Build history of the part. All positions in model axes, mm. A direction names the side the tool comes from. Give positions to 0.01 mm unless a question says otherwise; leave off trailing zeros. Order: outer loops, then holes, each group sorted by start corner. A loop starts at its lowest first (then second) coordinate and runs counter-clockwise, first axis right, second up. Notation, with made-up numbers: (41, 25) - (100, 25) arc R32 ccw to (100, 62) - close; hole circle Ø1 at (-38, 74). An arc over 180 degrees is marked (long way). One line per item, written item: value.
```python
from build123d import *

# Parameters (mm, degrees)
BOSS_EXTRUDE1_DEPTH     = 21.5
BOSS_EXTRUDE2_DEPTH     = 6
CHAMFER1_SIZE           = 1.5
SKETCH2_W               = 4.6
SKETCH2_H               = 18
CUT_EXTRUDE1_DEPTH      = 4.5000001
CUT_EXTRUDE1_DEPTH_BACK = 4.5000001
SKETCH3_R               = 1.6
CUT_EXTRUDE2_DEPTH      = 16
CHAMFER2_SIZE           = 0.5
SKETCH4_R               = 1.6
CUT_EXTRUDE3_DEPTH      = 7.0000001
CUT_EXTRUDE3_DEPTH_BACK = 7.0000001
SKETCH6_R               = 3
CUT_EXTRUDE4_DEPTH      = 2
CUT_EXTRUDE5_DEPTH      = 2
BOSS_EXTRUDE3_START     = -4.1
SKETCH8_R               = 1.6
BOSS_EXTRUDE3_DEPTH     = 3.5
BOSS_EXTRUDE4_DEPTH     = 9
BOSS_EXTRUDE5_DEPTH     = 9
CUT_EXTRUDE6_DEPTH      = 2
SKETCH13_W              = 5.8
SKETCH13_H              = 3
CUT_EXTRUDE8_DEPTH      = 18.5


with BuildPart() as part:
    # Sketch1 → Boss-Extrude1 (new body, symmetric)
    with BuildSketch(Plane.XY):
        with BuildLine():
            Line((-4.873397172, 3.5), (4.873397172, 3.5))
            ThreePointArc((4.873397172, 3.5), (6, 0), (4.873397172, -3.5))
            Line((4.873397172, -3.5), (-4.873397172, -3.5))
            ThreePointArc((-4.873397172, -3.5), (-6, 0), (-4.873397172, 3.5))
        make_face()
    extrude(amount=BOSS_EXTRUDE1_DEPTH, both=True)

    # Sketch5 → Boss-Extrude2 (add, symmetric)
    with BuildSketch(Plane(origin=(0, 0, 0), x_dir=(0, 0, -1), z_dir=(1, 0, 0))):
        with BuildLine():
            Line((-1.936491673, 3.5), (1.936491673, 3.5))
            ThreePointArc((1.936491673, 3.5), (4, 0), (1.936491673, -3.5))
            Line((1.936491673, -3.5), (-1.936491673, -3.5))
            ThreePointArc((-1.936491673, -3.5), (-4, 0), (-1.936491673, 3.5))
        make_face()
    extrude(amount=BOSS_EXTRUDE2_DEPTH, both=True)

    # Chamfer1
    chamfer1_edges = [part.edges().sort_by_distance(p)[0] for p in [
        (-6, 0, 21.5),
        (6, 0, 21.5),
        (-6, 0, -21.5),
        (6, 0, -21.5),
    ]]
    chamfer(chamfer1_edges, length=CHAMFER1_SIZE)

    # Sketch2 → Cut-Extrude1 (cut, two sides)
    with BuildSketch(Plane(origin=(0, 0, 0), x_dir=(1, 0, 0), z_dir=(0, 1, 0))) as cut_extrude1_sk:
        Rectangle(SKETCH2_W, SKETCH2_H)
    extrude(amount=CUT_EXTRUDE1_DEPTH, mode=Mode.SUBTRACT)
    extrude(cut_extrude1_sk.sketch, amount=-CUT_EXTRUDE1_DEPTH_BACK, mode=Mode.SUBTRACT)

    # Sketch3 → Cut-Extrude2 (cut)
    with BuildSketch(Plane.XY.offset(21.5)):
        Circle(SKETCH3_R)
    cut_extrude2 = extrude(amount=-CUT_EXTRUDE2_DEPTH, mode=Mode.SUBTRACT)

    # Mirror2: Cut-Extrude2 across plane
    add(cut_extrude2.mirror(Plane.XY), mode=Mode.SUBTRACT)

    # Chamfer2
    chamfer2_edges = [part.edges().sort_by_distance(p)[0] for p in [
        (-1.6, 0, 21.5),
        (-1.6, 0, -21.5),
    ]]
    chamfer(chamfer2_edges, length=CHAMFER2_SIZE)

    # Sketch4 → Cut-Extrude3 (cut, two sides)
    with BuildSketch(Plane(origin=(0, 0, 0), x_dir=(0, 0, -1), z_dir=(1, 0, 0))) as cut_extrude3_sk:
        Circle(SKETCH4_R)
    extrude(amount=CUT_EXTRUDE3_DEPTH, mode=Mode.SUBTRACT)
    extrude(cut_extrude3_sk.sketch, amount=-CUT_EXTRUDE3_DEPTH_BACK, mode=Mode.SUBTRACT)

    # Sketch6 → Cut-Extrude4 (cut)
    with BuildSketch(Plane(origin=(6, 0, 0), x_dir=(0, 0, -1), z_dir=(1, 0, 0))):
        Circle(SKETCH6_R)
    extrude(amount=-CUT_EXTRUDE4_DEPTH, mode=Mode.SUBTRACT)

    # Sketch7 → Cut-Extrude5 (cut)
    with BuildSketch(Plane.ZY.offset(6)):
        Polygon((3.233161507, 0), (1.616580754, 2.8), (-1.616580754, 2.8), (-3.233161507, 0), (-1.616580754, -2.8), (1.616580754, -2.8), align=None)
    extrude(amount=-CUT_EXTRUDE5_DEPTH, mode=Mode.SUBTRACT)

    # Sketch8 → Boss-Extrude3 (add)
    with BuildSketch(Plane(origin=(0, 0, 0), x_dir=(0, 0, -1), z_dir=(1, 0, 0)).offset(BOSS_EXTRUDE3_START)):
        with BuildLine():
            Line((-19.5, 9.5), (-19.5, 1))
            Line((-19.5, 1), (-10.5, 1))
            Line((-10.5, 1), (-10.5, 9.5))
            ThreePointArc((-10.5, 9.5), (-15, 14), (-19.5, 9.5))
        make_face()
        with Locations((-15, 9.5)):
            Circle(SKETCH8_R, mode=Mode.SUBTRACT)
    extrude(amount=-BOSS_EXTRUDE3_DEPTH)

    # Sketch9 → Boss-Extrude4 (add)
    with BuildSketch(Plane.XY.offset(19.5)):
        Polygon((-7.6, 1), (-4.1, 1), (-4.873397172, -3.5), align=None)
    extrude(amount=-BOSS_EXTRUDE4_DEPTH)

    # Sketch10 → Boss-Extrude5 (add)
    with BuildSketch(Plane.XY.offset(19.5)):
        Polygon((-4.1, 4.5), (-3.1, 3.5), (-4.1, 3.5), align=None)
    extrude(amount=-BOSS_EXTRUDE5_DEPTH)

    # Sketch11 → Cut-Extrude6 (cut)
    with BuildSketch(Plane.ZY.offset(7.6)):
        Polygon((15, 6.151368439), (17.9, 7.825684219), (17.9, 11.174315781), (15, 12.848631561), (12.1, 11.174315781), (12.1, 7.825684219), align=None)
    extrude(amount=-CUT_EXTRUDE6_DEPTH, mode=Mode.SUBTRACT)

    # Sketch13 → Cut-Extrude8 (cut, through all)
    with BuildSketch(Plane.XZ.offset(3.5)):
        with Locations((0, 14.5)):
            Rectangle(SKETCH13_W, SKETCH13_H)
    cut_extrude8 = extrude(amount=-CUT_EXTRUDE8_DEPTH, mode=Mode.SUBTRACT)

    # Mirror4: Cut-Extrude8 across plane
    add(cut_extrude8.mirror(Plane.XY), mode=Mode.SUBTRACT)


solid = part.part
```
(1) 3-axis set-ups, long thin cutter, end or side, ignore diameter. For faces 4 (the face through (-5.679, -2.804, 2.852)), 5 (the face through (2.9, 0, -14)), 6 (the face through (-5.679, 2.762, 2.894)), 7 (the face through (-5.935, -0.88, 7.081)): which of +Z, -Z, +X, -X, +Y, -Y reach the whole face in a straight line?
Completed:
face 4: -X, -Y
face 5: +Y, -Y
face 6: -X, +Y
face 7: -X
(2) Pin check, flat tips, straight feed: P1, Ø2, axis at x = -6, y = 9.5, coming from the +Z side; P2, Ø3.5, axis at y = 0, z = 4, coming from the -X side; P3, Ø6, axis at x = 3.5, z = -5.5, coming from the +Y side. Stop position of each tip, or through.
Completed:
P1: z = 19.5
P2: x = -6
P3: y = 3.5
(3) Pull direction Y, two halves, no side cores. Call faces 1 (the face through (-1.27, -0.97, -18.54)), 2 (the face through (-3, -3.5, 0)), 3 (the face through (-6, 1, 3)): +Y half, -Y half, draft (parallel to the pull), parting line (faces both ways), or undercut.
Completed:
face 1: undercut
face 2: -Y half
face 3: draft
(4) Slice it at B-B, the plane y = 8.5. Give the cut face in (x, z), and give its area (3 significant figures).
Completed:
outline: (-7.6, 10.5) - (-4.1, 10.5) - (-4.1, 13.75) - (-5.6, 13.75) - (-5.6, 12.1) - (-7.6, 12.1) - close; (-7.6, 17.9) - (-5.6, 17.9) - (-5.6, 16.25) - (-4.1, 16.25) - (-4.1, 19.5) - (-7.6, 19.5) - close
area: 16.2 mm²
(5) Slice it at A-A, the plane z = 0. Give the cut face in (x, y), and give its area (3 significant figures).
Completed:
outline: (-6, -3.5) - (-2.3, -3.5) - (-2.3, -1.6) - (-4, -1.6) - (-4, -2.8) - (-6, -2.8) - close; (-6, 2.8) - (-4, 2.8) - (-4, 1.6) - (-2.3, 1.6) - (-2.3, 3.5) - (-6, 3.5) - close; (2.3, -3.5) - (6, -3.5) - (6, -3) - (4, -3) - (4, -1.6) - (2.3, -1.6) - close; (2.3, 1.6) - (4, 1.6) - (4, 3) - (6, 3) - (6, 3.5) - (2.3, 3.5) - close
area: 17.7 mm²
(6) Drill centre lines: line 1 (Y direction, x = 0, z = -19.1); line 2 (X direction, y = -2.5, z = -3); line 3 (Y direction, x = -4.5, z = 15). Where is each one in solid material? Low to high.
Completed:
line 1: -3.5 to -1.6, 1.6 to 3.5
line 2: -6 to -2.3, 2.3 to 6
line 3: -3.5 to 7.9, 11.1 to 14
(7) Slice it at C-C, the plane x = 0. Count the separate pieces of the cut face and the enclosed holes in it, and give its area (3 significant figures).
Completed:
separate pieces: 8
enclosed holes: 0
area: 71.7 mm²
